Answer from the drawing. Dimensions are ordinates in mm from the lowest x, y and z of the part. A direction names the side the tool comes from. Give positions to 0.01 mm unless a question says otherwise; leave off trailing zeros. Loops run counter-clockwise (first coordinate to the right, second up) from the corner with the lowest first, then second, coordinate; pieces in that order, holes last. Notation, with made-up numbers: M 29,33.25 L 70,33.25 A23 cw 70,56.25 Z; hole C 60,66 d5. An arc over 180 degrees is marked long. Return JSON: item names as keys, results as strings. Group by question number.
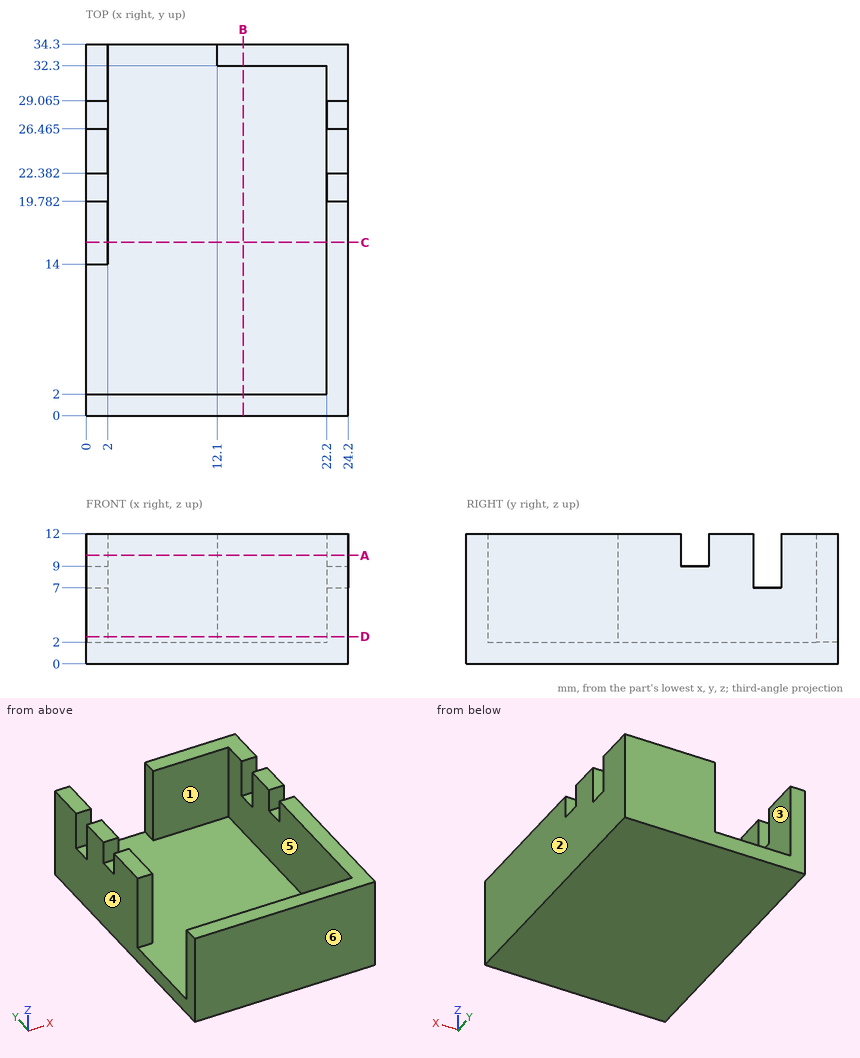
1. Find section C-C (y = 16). Write down the section's boundary in (x, z).
2. Find section A-A (z = 10). Write down the section's boundary in (x, y) (1 decimal).
3. Straight lines are drawn through the part: line 1 along Y through (x, z) = (21, 7.5); line 2 along X through (y, z) = (24, 6.25); line 3 along Y through (x, z) = (1, 4.75). For each, find the intervals that lie inside material, in ascending order.
4. For the marked faces 1, 2 and 3, determine the directions among +Z, -Z, +X, -X, +Y, -Y from which every point of the face is accessible in a straight line to the end or side of a thin tool.
5. The mould has two halves that part along Y. Classify the marked faces 4, 5 and 6: +Y half, -Y half, draft (parallel to the pull), parting line (faces both ways), or undercut.
6. Flat-ended cylindrical pins translate along their axes: P1, Ø2, axis at x = 1, z = 10.5, coming from the -Y side; P2, Ø2, axis at x = 17, y = 28.5, coming from the +Z side; P3, Ø0.6, axis at x = 1.5, y = 27.5, coming from the +Z side; P4, Ø3, axis at x = 9.5, z = 9.5, coming from the +Y side. Find the tip coordinate at first contact, or state that the pin passes through.
7. Find section B-B (x = 14.5). Write down the section's boundary in (y, z).
8. Find section D-D (z = 2.5). Write down the section's boundary in (x, y), and give its area (3 significant figures).
Result:
{
 "1": {"outline": "M 0,0 L 24.2,0 L 24.2,12 L 22.2,12 L 22.2,2 L 2,2 L 2,12 L 0,12 Z"},
 "2": {"outline": "M 0,0 L 24.2,0 L 24.2,19.8 L 22.2,19.8 L 22.2,2 L 0,2 Z; M 0,14 L 2,14 L 2,19.8 L 0,19.8 Z; M 0,22.4 L 2,22.4 L 2,26.5 L 0,26.5 Z; M 0,29.1 L 2,29.1 L 2,34.3 L 0,34.3 Z; M 12.1,32.3 L 22.2,32.3 L 22.2,29.1 L 24.2,29.1 L 24.2,34.3 L 12.1,34.3 Z; M 22.2,22.4 L 24.2,22.4 L 24.2,26.5 L 22.2,26.5 Z"},
 "3": {"line 1": "y = 0 to 2, 32.3 to 34.3", "line 2": "x = 0 to 2, 22.2 to 24.2", "line 3": "y = 0 to 2, 14 to 34.3"},
 "4": {"face 1": "+Z", "face 2": "+Z, -Z, +X, +Y, -Y", "face 3": "+Z, +Y"},
 "5": {"face 4": "draft", "face 5": "undercut", "face 6": "-Y half"},
 "6": {"P1": "stops at y = 0", "P2": "stops at z = 2", "P3": "stops at z = 7", "P4": "stops at y = 2"},
 "7": {"outline": "M 0,0 L 34.3,0 L 34.3,12 L 32.3,12 L 32.3,2 L 2,2 L 2,12 L 0,12 Z"},
 "8": {"outline": "M 0,0 L 24.2,0 L 24.2,34.3 L 12.1,34.3 L 12.1,32.3 L 22.2,32.3 L 22.2,2 L 0,2 Z; M 0,14 L 2,14 L 2,34.3 L 0,34.3 Z", "area": "174 mm2"}
}
